Geometry check sheet. Reference: the model listing, model coordinates, mm. A direction names the side the tool comes from. Coordinates: 2 decimals unless noted, no trailing zeros. Write each loop counter-clockwise with the first axis right and the second up, starting at its lowest first coordinate (ties: lowest second). Pieces come first, ordered by that corner, then holes. Notation, with made-up numbers: M 87,59 L 127,59 A28 ccw 127,84 Z; hole C -12.75,74.25 d7. An arc over 180 degrees is marked long. Write each question's results on one line, items separated by ' | '.
```python
from build123d import *

# Parameters (mm, degrees)
F0_W     = 41.5
F0_H     = 49
F1_DEPTH = 16.5
F2_W     = 39.5
F2_H     = 14.5
F3_DEPTH = 48
F4_W     = 8
F4_H     = 5.5
F5_DEPTH = 1.000984
F6_W     = 5.75
F6_H     = 22
F7_DEPTH = 3.5


with BuildPart() as f1:
    # F0 (on Top) → F1 (new body)
    with BuildSketch(Plane.XY):
        with Locations((-20.077741, -10.186185)):
            Rectangle(F0_W, F0_H)
    extrude(amount=F1_DEPTH)

    # F2 (on face) → F3 (cut)
    with BuildSketch(Plane(origin=(0, 14.313815, 0), x_dir=(-1, 0, 0), z_dir=(0, 1, 0))):
        with Locations((20.061721, 8.249016)):
            Rectangle(F2_W, F2_H)
    extrude(amount=-F3_DEPTH, mode=Mode.SUBTRACT)

    # F4 (on face) → F5 (cut, through all)
    with BuildSketch(Plane.XY.offset(16.5)):
        with Locations((-12.947741, 11.563815)):
            Rectangle(F4_W, F4_H)
    extrude(amount=-F5_DEPTH, mode=Mode.SUBTRACT)

    # F6 (on face) → F7 (cut)
    with BuildSketch(Plane(origin=(0, 0, 0), x_dir=(1, 0, 0), z_dir=(0, 0, -1))):
        with Locations((-2.202741, 20.486185)):
            Rectangle(F6_W, F6_H)
    extrude(amount=-F7_DEPTH, mode=Mode.SUBTRACT)


solid = f1.part
```
Q1. Scan lines: probe 1 along X at (y, z) = (-25, 4.75); probe 2 along Z at (x, y) = (-15, -22); probe 3 along Y at (x, z) = (-22, 8.25). Record each from-to range of solid material in increasing order.
Geometry check:
probe 1: x = -40.83 to -39.81, -0.31 to 0.67 | probe 2: z = 0 to 1, 15.5 to 16.5 | probe 3: y = -34.69 to -33.69
Q2. Mould release check, pull along X, two halves, no side actions. Record for faces 4 (the flat face through (-20, -10, 16.5)), 5 (the flat face through (-20, -9, 15.499)), 6 (the flat face through (-40.828, -11, 8)): pulls with the +X half, pulls with the -X half, needs draft (parallel to the pull), parting line crosses it, or undercut.
Geometry check:
face 4: needs draft | face 5: undercut | face 6: pulls with the -X half
Q3. Sectioned sample at C-C on z = 2. Record the cut outline in (x, y).
Geometry check:
outline: M -40.83,-34.69 L 0.67,-34.69 L 0.67,-31.49 L -0.31,-31.49 L -0.31,-33.69 L -39.81,-33.69 L -39.81,14.31 L -40.83,14.31 Z; M -0.31,-9.49 L 0.67,-9.49 L 0.67,14.31 L -0.31,14.31 Z
Q4. Depth check by flat-ended pin: P1, Ø0.8, axis at x = 0.5, y = -23, coming from the -Z side. Enter the tip coordinate at first touch or a pass-through.
Geometry check:
P1: stops at z = 3.5
Q5. Sectioned sample at A-A on x = -1.5. Record the cut outline in (y, z).
Geometry check:
outline: M -34.69,0 L -31.49,0 L -31.49,1 L -33.69,1 L -33.69,15.5 L 14.31,15.5 L 14.31,16.5 L -34.69,16.5 Z; M -9.49,0 L 14.31,0 L 14.31,1 L -9.49,1 Z
Q6. Sectioned sample at D-D on x = -30. Record the cut outline in (y, z), and give its area (4 significant figures).
Geometry check:
outline: M -34.69,0 L 14.31,0 L 14.31,1 L -33.69,1 L -33.69,15.5 L 14.31,15.5 L 14.31,16.5 L -34.69,16.5 Z | area: 112.5 mm2
Q7. Sectioned sample at B-B on y = 7. Record the cut outline in (x, z).
Geometry check:
outline: M -40.83,0 L 0.67,0 L 0.67,16.5 L -40.83,16.5 Z; hole M -39.81,1 L -0.31,1 L -0.31,15.5 L -39.81,15.5 Z
Q8. Access from +Z, -Z, +X, -X, +Y, -Y to the whole of each face (thin tool, end or side, straight path). Record for faces 1 (the flat face through (-5.078, -20.3, 0.5)), 2 (the flat face through (-0.312, -9, 8)), 3 (the flat face through (-8.948, 12, 16)).
Geometry check:
face 1: -Z, +X | face 2: +Y | face 3: +Z, +Y
